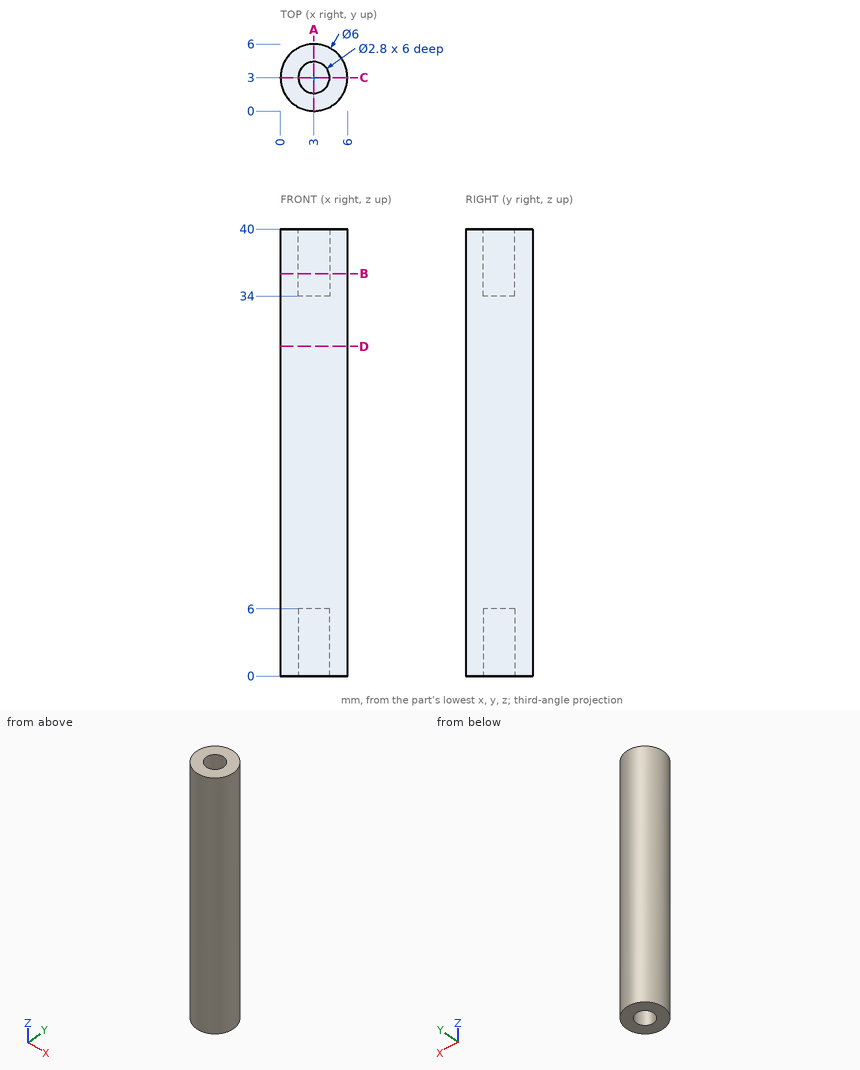
Source: three-view drawing plus pictorial views. Frame: mm from the lowest corner of the part. Give positions to 0.01 mm unless a question says otherwise; leave off trailing zeros. Order: outer loops, then holes, each group sorted by start corner. A loop starts at its lowest first (then second) coordinate and runs counter-clockwise, first axis right, second up. Notation, with made-up numbers: (76.25, 7.25) - (120.25, 7.25) arc R19 ccw to (120.25, 29.25) - close; hole circle Ø2 at (36, 15.25). An arc over 180 degrees is marked (long way). Put each result on its own line as item: value.
Item 1: Ray query, L1, parallel to Y at x = 3, z = 38.6; L2, parallel to Z at x = 2.6, y = 3.75; L3, parallel to X at y = 0.55, z = 14. Return the intervals inside material, ascending. Write a range as from..to.
Found:
L1: y = 0..1.6, 4.4..6
L2: z = 6..34
L3: x = 1.27..4.73
Item 2: Section query B-B, the plane z = 36. Return loops of the section in (x, y).
Found:
outline: circle Ø6 at (3, 3); hole circle Ø2.8 at (3, 3)
Item 3: Section query D-D, the plane z = 29.5. Return loops of the section in (x, y), then the cut area to 3 significant figures.
Found:
outline: circle Ø6 at (3, 3)
area: 28.3 mm^2
Item 4: Contact query for flat-ended pins moving along their axis: pin 1 (2 mm diameter, centred on x = 5, z = 18, fed in from -Y); pin 2 (3 mm diameter, centred on y = 0.5, z = 25, fed in from +X); pin 3 (1 mm diameter, centred on y = 0.5, z = 15, fed in from -X). Output: stop coordinate, or through.
Found:
pin 1: stops at y = 0.17
pin 2: stops at x = 5.83
pin 3: stops at x = 0.76
Item 5: Section query A-A, the plane x = 3. Return loops of the section in (y, z), then the cut area to 3 significant figures.
Found:
outline: (0, 0) - (1.6, 0) - (1.6, 6) - (4.4, 6) - (4.4, 0) - (6, 0) - (6, 40) - (4.4, 40) - (4.4, 34) - (1.6, 34) - (1.6, 40) - (0, 40) - close
area: 206 mm^2
